Can you work these out from the model? Positions are in its coordinate system, mm. Face numbers are marked on the shaded views. A direction names the side the tool comes from. Give positions to 0.01 mm unless a question says otherwise; leave off trailing zeros. Order: outer loops, then holes, each group sorted by start corner. A loop starts at its lowest first (then second) coordinate and runs counter-clockwise, first axis right, second up. Notation, with made-up numbers: (0.5, -3) -> (51.5, -3) arc R20 ccw to (51.5, 27) -> close; hole circle Ø6 at (16, -16.75). An arc over 180 degrees is marked (long way). Answer as a JSON object with one key per item and string values.
Autodesk Inventor part; units mm, degrees
ref_plane "YZ Plane" through (0, 0, 0) normal (1, 0, 0) x (0, 1, 0)
ref_plane "XZ Plane" through (0, 0, 0) normal (0, 1, 0) x (-1, 0, 0)
ref_plane "XY Plane" through (0, 0, 0) normal (0, 0, 1) x (1, 0, 0)
sketch "Sketch2" plane through (0, 0, 0) normal (0, 0, 1) x (1, 0, 0)
  circle A0 centre (0, 0) radius 11
  dimension "d1" = 22
extrude "Extrusion1" add sketch "Sketch2" along normal blind 65
sketch "Sketch3" plane through (0, 0, 65) normal (0, 0, 1) x (1, 0, 0)
  circle A0 centre (0, 0) radius 6
  dimension "d4" = 12
extrude "Extrusion2" cut sketch "Sketch3" against normal blind 40
thread "Thread1"
sketch "Sketch6" plane through (0, 0, 0) normal (0, 1, 0) x (-1, 0, 0)
  line L0 (11, 65) -> (-11, 65) construction
  line L1 (-11.5, -5) -> (56.1068, -5) construction
  line L2 (0, 0) -> (0, -163.2122) construction
  line L3 (8.5, -107.4374) -> (8.5, -5) construction
  line L4 (18.5, -103.8042) -> (18.5, -5) construction
  circle A0 centre (8.5, -5) radius 15
  line L5 (-11.5, -59.4325) -> (-11.5, -5) construction
  circle A1 centre (8.5, -5) radius 20 construction
  line L6 (18.5, -30) -> (18.5, 20) construction
  line L7 (18.5, -30) -> (-11.5, -18.9445) construction
  line L8 (22.2477, -5) -> (22.2477, -11) construction
  line L9 (22.2477, -11) -> (58.2477, -11)
  line L10 (58.2477, -11) -> (58.2477, -5)
  line L11 (23.5, -5) -> (58.2477, -5)
  line L12 (18.5, -30) -> (-11.5, -30) construction
  line L13 (18.5, -25) -> (-11.5, -25) construction
  line L14 (8.5, -20) -> (8.5, -25)
  line L15 (8.5, -25) -> (18.5, -25)
  line L16 (18.5, -25) -> (18.5, -30)
  line L17 (18.5, -30) -> (0, -30)
  arc A2 (-11.5, -5) -> (8.5, -30) centre (14.125, -5) ccw
  line L18 (-11.5, -5) -> (-6.5, -5)
  line L19 (23.5, -5) -> (-6.5, -5)
  point P0 (18.5, -5)
  dimension "d27" = 70
  dimension "d28" = 8.5
  dimension "d30" = 30
  dimension "d31" = 30
  dimension "d32" = 5
  dimension "d33" = 50
  dimension "d34" = 6
  dimension "d35" = 36
  dimension "d36" = 5
  dimension "d37" = 10
revolve "Revolution2" add sketch "Sketch6" angle 360 about axis through (11.5, 0, -5) along (-1, 0, 0) contours A0 L14 L15 L16 L17 A2 L18
sketch "Sketch7" plane through (0, 0, 0) normal (0, 1, 0) x (-1, 0, 0)
  line L0 (23.5, -5) -> (-6.5, -5)
  line L1 (18.5, -30) -> (18.5, 20) construction
  line L2 (18.5, -25) -> (-11.5, -25) construction
  line L3 (8.5, -107.4374) -> (8.5, -5) construction
  line L4 (18.5, -5) -> (18.5, -25)
  line L5 (8.5, -25) -> (8.5, -5)
  line L6 (8.5, -5) -> (18.5, -5)
  line L7 (18.5, -25) -> (8.5, -25)
  point P0 (0, 0)
thread "Thread2"
revolve "Revolution6" cut sketch "Sketch6" angle 360 about axis through (11.5, 0, -5) along (-1, 0, 0) picked at (6.409, -11.3012) contours A0 L19
revolve "Revolution7" cut sketch "Sketch7" angle 360 about axis through (-23.5, 0, -5) along (1, 0, 0)
equation "\"d4\" = Screw_DIA"
equation "\"d5\" = ScrewDEPTH"
equation "\"d16\" = 55deg"
equation "\"Sketch4_Pitch\" = 1.25"
equation "\"d50\" = 55deg"
equation "\"Sketch8_Pitch\" = 1.5"
properties part number "MCEN4000:T4" material "STEEL, AISI 1040"
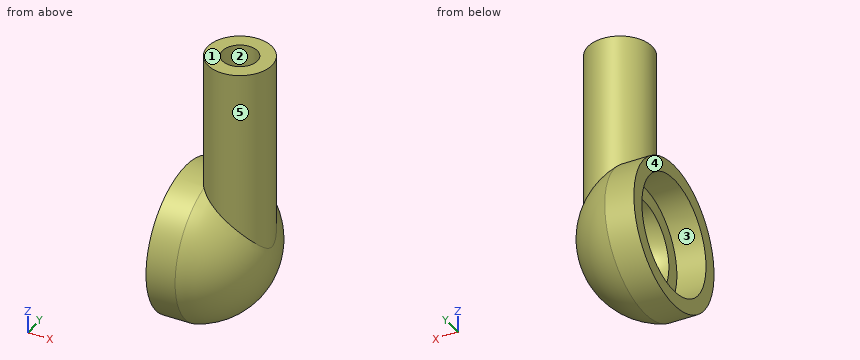
1. If we mould it in two halves opening along Y, with no side actions, what happens to the marked faces 3, 4 and 5? For each: +Y half, -Y half, draft (parallel to the pull), parting line (faces both ways), or undercut.
Worked answers:
{"face 3": "undercut", "face 4": "draft", "face 5": "parting line"}
2. If we section it at B-B on z = -5: Please give me the cut outline in (x, y) (3 decimals), then the cut area to 3 significant figures.
Worked answers:
{"outline": "(-18.5, -25) -> (-8.5, -25) arc R25.625 ccw to (-8.5, 25) -> (-18.5, 25) -> (-18.5, 20) -> (-8.5, 20) -> (-8.5, 15) arc R15 cw to (-8.5, -15) -> (-8.5, -20) -> (-18.5, -20) -> close", "area": "492 mm²"}
3. Will these pins go through, and if not, where does the flat tip stop? pin 1 Ø8 at (y, z) = (-13.5, 42) entering from -X; pin 2 Ø8 at (x, y) = (0, -13.5) entering from -Z; pin 3 Ø4 at (x, y) = (-3.5, 11.5) entering from +Z; pin 4 Ø9.5 at (x, y) = (-0.5, 0.5) entering from +Z.
Worked answers:
{"pin 1": "x = -5.55", "pin 2": "z = -25.38", "pin 3": "z = 65", "pin 4": "z = 25"}
4. If we section it at A-A on y = 0: Please give me the cut outline in (x, z) (3 decimals), then the cut area to 3 significant figures.
Worked answers:
{"outline": "(-18.5, -30) -> (-8.5, -30) arc R25.625 ccw to (11, 0.037) -> (11, 65) -> (6, 65) -> (6, 25) -> (-6, 25) -> (-6, 65) -> (-11, 65) -> (-11, 20) -> (-18.5, 20) -> (-18.5, 15) -> (-8.5, 15) -> (-8.5, 10) arc R15 cw to (-8.5, -20) -> (-8.5, -25) -> (-18.5, -25) -> close", "area": "1,120 mm²"}
5. For the marked faces 1 and 2, which set-ups out of +Z, -Z, +X, -X, +Y, -Y let a thin tool reach every point of the face, with its end or its side?
Worked answers:
{"face 1": "+Z, +X, -X, +Y, -Y", "face 2": "+Z"}
6. Please list where these lines run through material, in increasing order: L1, parallel to Z at x = -12, y = 0; L2, parallel to Y at x = 0, z = 51; L3, parallel to Y at x = -13.5, z = -5.
Worked answers:
{"L1": "-30 to -25, 15 to 20", "L2": "-11 to -6, 6 to 11", "L3": "-25 to -20, 20 to 25"}
7. If we section it at C-C on x = 4: Please give me the cut outline in (y, z).
Worked answers:
{"outline": "(-10.25, 9.94) arc R18.11 ccw (long way) to (10.25, 9.94) -> (10.25, 65) -> (4.47, 65) -> (4.47, 25) -> (-4.47, 25) -> (-4.47, 65) -> (-10.25, 65) -> close; hole circle Ø16.58 at (0, -5)"}
8. If we section it at D-D on z = 59: Please give me the cut outline in (x, y), then the cut area to 3 significant figures.
Worked answers:
{"outline": "circle Ø22 at (0, 0); hole circle Ø12 at (0, 0)", "area": "267 mm²"}
